from build123d import *

# Parameters (mm, degrees)
SKETCH1_W           = 125
SKETCH1_H           = 125
BOSS_EXTRUDE1_DEPTH = 100
FILLET1_R           = 50


with BuildPart() as part:
    # Sketch1 → Boss-Extrude1 (new body)
    with BuildSketch(Plane.XY):
        with Locations((62.5, 62.5)):
            Rectangle(SKETCH1_W, SKETCH1_H)
    extrude(amount=BOSS_EXTRUDE1_DEPTH)

    # Fillet1
    fillet1_edges = [part.edges().sort_by_distance(p)[0] for p in [
        (62.5, 0, 0),
        (125, 62.5, 0),
        (62.5, 125, 0),
        (0, 62.5, 0),
        (62.5, 125, 100),
        (125, 62.5, 100),
        (62.5, 0, 100),
        (0, 62.5, 100),
    ]]
    fillet(fillet1_edges, radius=FILLET1_R - 0.0001)  # a hair under: the kernel refuses the full size


solid = part.part
Build history of the part. All positions in model axes, mm. Round coordinates to 2 decimals unless told otherwise and drop trailing zeros. Write each loop counter-clockwise with the first axis right and the second up, starting at its lowest first coordinate (ties: lowest second). Pieces come first, ordered by that corner, then holes. Notation, with made-up numbers: (-11.75, 20.25) - (-1.75, 20.25) arc R16 cw to (-1.75, 38.25) - close; hole circle Ø6 at (-25.5, -32). An arc over 180 degrees is marked (long way). One line per question, with ' | ' between items.
1. Band-saw the part on D-D, the plane z = 87.5. Write the cut outline in (x, y), and give its area (3 significant figures).
Results are:
outline: (16.93, 16.93) - (108.07, 16.93) - (108.07, 108.07) - (16.93, 108.07) - close | area: 8,310 mm^2
2. Drill centre lines: line 1 along Z through (x, y) = (53, 76); line 2 along Y through (x, z) = (24.5, 54); line 3 along Z through (x, y) = (113, 92). Where is each one in solid material? Low to high. Write a range as from..to.
Results are:
line 1: 0.01..99.99 | line 2: 0.16..124.84 | line 3: 17.5..82.5
3. Band-saw the part on C-C, the plane z = 64. Write the cut outline in (x, y), and give its area (3 significant figures).
Results are:
outline: (2, 2) - (123, 2) - (123, 123) - (2, 123) - close | area: 14,600 mm^2
4. Drop flat-ended pins along their axis: pin 1 Ø6 at (y, z) = (90.5, 27) entering from -X; pin 2 Ø5 at (x, y) = (47, 15.5) entering from -Z; pin 3 Ø5 at (x, z) = (78, 41) entering from +Y. Give the stop position or say it passes through.
Results are:
pin 1: x = 4.17 | pin 2: z = 11.58 | pin 3: y = 124.58
